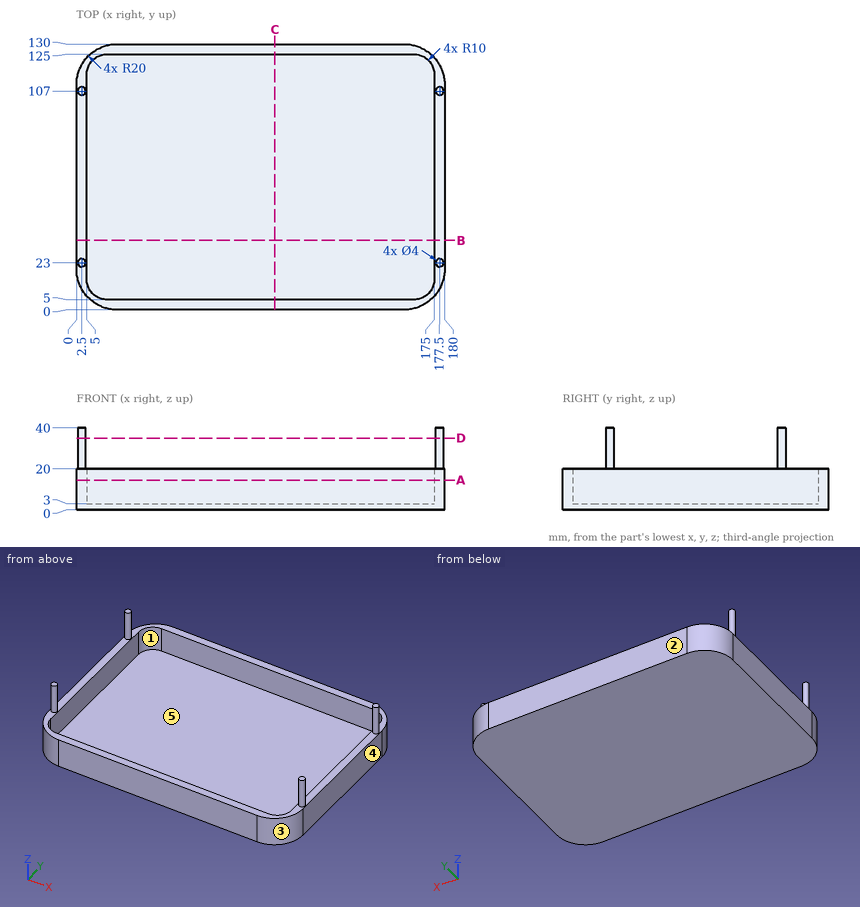
Could you check a few things on this drawing? It's one solid part, dimensions in mm from its lowest x, y, z. A direction names the side the tool comes from. Round coordinates to 2 decimals unless told otherwise and drop trailing zeros. Loops run counter-clockwise (first coordinate to the right, second up) from the corner with the lowest first, then second, coordinate; pieces in that order, holes last. Notation, with made-up numbers: (87.5, 53) -> (130.5, 53) arc R23 ccw to (130.5, 90) -> close; hole circle Ø2 at (59, 65.5). An arc over 180 degrees is marked (long way). Write each question's results on one line, items separated by ' | '.
(1) We'd pull the mould along X, two halves only. Please class the marked faces 1, 2 and 3: released by +X, released by -X, zero draft, split by the parting line, or undercut.
Worked answers:
face 1: undercut | face 2: zero draft | face 3: released by +X
(2) If we section it at D-D, the plane z = 35: List the corners of the cut face in (x, y) for me, then the cut area to 3 significant figures.
Worked answers:
outline: circle Ø4 at (2.5, 23); circle Ø4 at (2.5, 107); circle Ø4 at (177.5, 23); circle Ø4 at (177.5, 107) | area: 50.3 mm2
(3) For P1, Ø6, axis at x = 40.5, y = 85.5, coming from the +Z side, with a flat end and sliding along its axis, tell me the tip position at first contact or that it passes through.
Worked answers:
P1: z = 3
(4) If we section it at A-A, the plane z = 14.5: List the corners of the cut face in (x, y) for me.
Worked answers:
outline: (0, 20) arc R20 ccw to (20, 0) -> (160, 0) arc R20 ccw to (180, 20) -> (180, 110) arc R20 ccw to (160, 130) -> (20, 130) arc R20 ccw to (0, 110) -> close; hole (5, 15) arc R10 ccw to (15, 5) -> (165, 5) arc R10 ccw to (175, 15) -> (175, 115) arc R10 ccw to (165, 125) -> (15, 125) arc R10 ccw to (5, 115) -> close
(5) If we section it at B-B, the plane y = 34: List the corners of the cut face in (x, z) for me, then the cut area to 3 significant figures.
Worked answers:
outline: (0, 0) -> (180, 0) -> (180, 20) -> (175, 20) -> (175, 3) -> (5, 3) -> (5, 20) -> (0, 20) -> close | area: 710 mm2
(6) If we section it at C-C, the plane x = 97: List the corners of the cut face in (y, z) for me, then the cut area to 3 significant figures.
Worked answers:
outline: (0, 0) -> (130, 0) -> (130, 20) -> (125, 20) -> (125, 3) -> (5, 3) -> (5, 20) -> (0, 20) -> close | area: 560 mm2
(7) If I drill on L1, parallel to Y at x = 32, z = 18; L2, parallel to X at y = 43.5, z = 6; L3, parallel to Z at x = 88.5, y = 17.5, over which ranges is the centre line in solid material (lowest first)?
Worked answers:
L1: 0 to 5, 125 to 130 | L2: 0 to 5, 175 to 180 | L3: 0 to 3
(8) For the marked faces 4 and 5, which set-ups out of +Z, -Z, +X, -X, +Y, -Y let a thin tool reach every point of the face, with its end or its side?
Worked answers:
face 4: +Z, -Z, +X, +Y, -Y | face 5: +Z
